from build123d import *

# Parameters (mm, degrees)
SKETCH_1_R          = 15
EXTRUDE_1_DEPTH     = 10
SKETCH_2_R          = 5.995
EXTRUDE_2_DEPTH     = 5
SKETCH_3_R          = 6.495
EXTRUDE_3_DEPTH     = 0.5
SKETCH_4_R          = 1.65
CUT_EXTRUDE_1_DEPTH = 10
SKETCH_5_R          = 2.15
CUT_EXTRUDE_2_DEPTH = 15


with BuildPart() as part:
    # ｽｹｯﾁ1 → ﾎﾞｽ - 押し出し1 (new body)
    with BuildSketch(Plane(origin=(0, 0, 0), x_dir=(1, 0, 0), z_dir=(0, 1, 0))):
        with Locations(Location((0, 0, 0), (0, 0, 270))):
            Circle(SKETCH_1_R)
    extrude(amount=EXTRUDE_1_DEPTH)

    # ｽｹｯﾁ2 → ﾎﾞｽ - 押し出し2 (add)
    with BuildSketch(Plane(origin=(0, 10, 0), x_dir=(1, 0, 0), z_dir=(0, 1, 0))):
        with Locations(Location((0, 0, 0), (0, 0, 270))):
            Circle(SKETCH_2_R)
    extrude(amount=EXTRUDE_2_DEPTH)

    # ｽｹｯﾁ3 → ﾎﾞｽ - 押し出し3 (add)
    with BuildSketch(Plane(origin=(0, 10, 0), x_dir=(1, 0, 0), z_dir=(0, 1, 0))):
        with Locations(Location((0, 0, 0), (0, 0, 270))):
            Circle(SKETCH_3_R)
    extrude(amount=EXTRUDE_3_DEPTH)

    # ｽｹｯﾁ4 → ｶｯﾄ - 押し出し1 (cut)
    with BuildSketch(Plane(origin=(0, 10, 0), x_dir=(1, 0, 0), z_dir=(0, 1, 0))):
        with Locations(Location((10, 0, 0), (0, 0, 270))):
            Circle(SKETCH_4_R)
        with Locations(Location((-10, 0, 0), (0, 0, 270))):
            Circle(SKETCH_4_R)
    extrude(amount=-CUT_EXTRUDE_1_DEPTH, mode=Mode.SUBTRACT)

    # ｽｹｯﾁ5 → ｶｯﾄ - 押し出し2 (cut)
    with BuildSketch(Plane(origin=(0, 15, 0), x_dir=(1, 0, 0), z_dir=(0, 1, 0))):
        with Locations(Location((0, 0, 0), (0, 0, 270))):
            Circle(SKETCH_5_R)
    extrude(amount=-CUT_EXTRUDE_2_DEPTH, mode=Mode.SUBTRACT)


solid = part.part
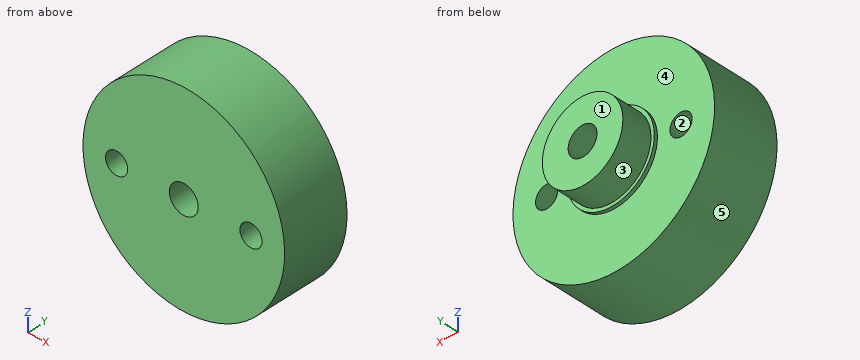
Could you check a few things on this model? Use its own coordinates, in mm. Face numbers are marked on the shaded views. A direction names the side the tool comes from. Give positions to 0.01 mm unless a question says otherwise; leave off trailing zeros. Order: outer loops, then holes, each group sorted by start corner. A loop starts at its lowest first (then second) coordinate and runs counter-clockwise, first axis right, second up. Notation, with made-up numbers: (47, 51.5) - (92, 51.5) arc R27 ccw to (92, 67.5) - close; hole circle Ø1 at (-16, -33.75). An arc over 180 degrees is marked (long way). One line per question, with ' | ' between items. Start each with the question number.
Item 1: I want a section at A-A on x = 0. Write out the boundary of the cut face in (y, z) (3 decimals).
Item 2: I need wall thicknesses on probe 1 along X at (y, z) = (7, 0); probe 2 along Y at (x, z) = (-11, 4.5); probe 3 along X at (y, z) = (4, -1.75). Which ranges of each line are inside material? Lowest first, please. Write a range as [from, to].
Item 3: I want a section at C-C on y = 12.5. Write out the boundary of the cut face in (x, z) (3 decimals).
Item 4: I want a section at D-D on z = -12. Write out the boundary of the cut face in (x, y).
Item 5: I want a section at B-B on z = 0. Write out the boundary of the cut face in (x, y) (3 decimals), then the cut area to 3 significant figures.
Item 6: Thinking about a two-plate mould opening in Z: for the marked faces 1, 2 and 3, which applies, pulls with the +Z half, pulls with the -Z half, needs draft (parallel to the pull), parting line crosses it, or undercut?
Item 7: I'm going to push flat-ended pins straight in: pin 1 Ø2 at (x, z) = (0.5, 1) entering from -Y; pin 2 Ø1 at (x, y) = (-7.5, 7) entering from +Z; pin 3 Ø6 at (y, z) = (7.5, -4) entering from -X; pin 4 Ø1.5 at (x, z) = (-11, 6.5) entering from +Y. Where does each tip first touch, or does it pass through?
Item 8: For the marked faces 4 and 5, which set-ups out of +Z, -Z, +X, -X, +Y, -Y let a thin tool reach every point of the face, with its end or its side?
Verdict:
1) outline: (0, -15) - (10, -15) - (10, -6.495) - (10.5, -6.495) - (10.5, -5.995) - (15, -5.995) - (15, -2.15) - (0, -2.15) - close; (0, 2.15) - (15, 2.15) - (15, 5.995) - (10.5, 5.995) - (10.5, 6.495) - (10, 6.495) - (10, 15) - (0, 15) - close
2) probe 1: [-15, -11.65], [-8.35, -2.15], [2.15, 8.35], [11.65, 15] | probe 2: [0, 10] | probe 3: [-14.9, -1.25], [1.25, 14.9]
3) outline: circle Ø11.99 at (0, 0); hole circle Ø4.3 at (0, 0)
4) outline: (-9, 0) - (9, 0) - (9, 10) - (-9, 10) - close
5) outline: (-15, 0) - (-11.65, 0) - (-11.65, 10) - (-15, 10) - close; (-8.35, 0) - (-2.15, 0) - (-2.15, 15) - (-5.995, 15) - (-5.995, 10.5) - (-6.495, 10.5) - (-6.495, 10) - (-8.35, 10) - close; (2.15, 0) - (8.35, 0) - (8.35, 10) - (6.495, 10) - (6.495, 10.5) - (5.995, 10.5) - (5.995, 15) - (2.15, 15) - close; (11.65, 0) - (15, 0) - (15, 10) - (11.65, 10) - close | area: 230 mm^2
6) face 1: needs draft | face 2: undercut | face 3: parting line crosses it
7) pin 1: through | pin 2: z = 13.27 | pin 3: x = -14.97 | pin 4: y = 10
8) face 4: +Y | face 5: +Y, -Y
